For this review, take the finished solid that the model builds, in its own axes (mm). Round coordinates to 2 decimals unless told otherwise and drop trailing zeros. Use a Markdown table: item, result.
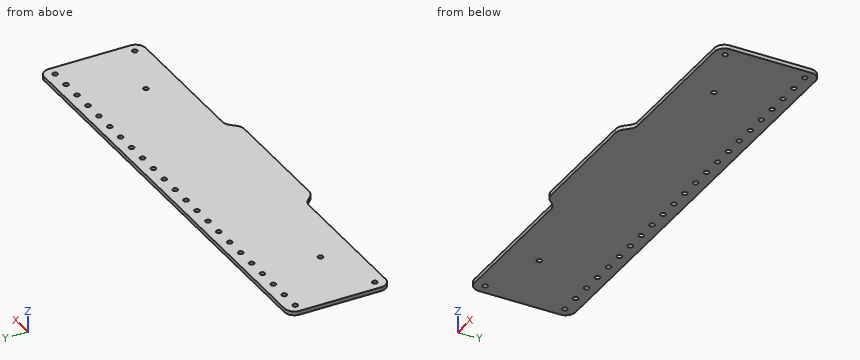
from build123d import *

# Parameters (mm, degrees)
SKETCH1_W           = 368
SKETCH1_H           = 90.35
SKETCH1_R           = 2.05
BOSS_EXTRUDE1_DEPTH = 3.175
SKETCH3_R           = 2.05
CUT_EXTRUDE1_DEPTH  = 3.18
CUT_EXTRUDE2_DEPTH  = 10
FILLET1_R           = 8


with BuildPart() as part:
    # Sketch1 → Boss-Extrude1 (new body)
    with BuildSketch(Plane.XY):
        Rectangle(SKETCH1_W, SKETCH1_H)
        with Locations((-128, -10.175)):
            Circle(SKETCH1_R, mode=Mode.SUBTRACT)
        with Locations(Location((128, -10.175, 0), (0, 0, 180))):
            Circle(SKETCH1_R, mode=Mode.SUBTRACT)
    extrude(amount=BOSS_EXTRUDE1_DEPTH)

    # Sketch3 → Cut-Extrude1 (cut)
    with BuildSketch(Plane.XY.offset(3.175)):
        with Locations((-176, 36.5)):
            Circle(SKETCH3_R)
        with Locations((-160, 36.5)):
            Circle(SKETCH3_R)
        with Locations((-144, 36.5)):
            Circle(SKETCH3_R)
        with Locations((-128, 36.5)):
            Circle(SKETCH3_R)
        with Locations((-112, 36.5)):
            Circle(SKETCH3_R)
        with Locations((-96, 36.5)):
            Circle(SKETCH3_R)
        with Locations((-80, 36.5)):
            Circle(SKETCH3_R)
        with Locations((-64, 36.5)):
            Circle(SKETCH3_R)
        with Locations((-48, 36.5)):
            Circle(SKETCH3_R)
        with Locations((-32, 36.5)):
            Circle(SKETCH3_R)
        with Locations((-16, 36.5)):
            Circle(SKETCH3_R)
        with Locations((0, 36.5)):
            Circle(SKETCH3_R)
        with Locations((16, 36.5)):
            Circle(SKETCH3_R)
        with Locations((32, 36.5)):
            Circle(SKETCH3_R)
        with Locations((48, 36.5)):
            Circle(SKETCH3_R)
        with Locations((64, 36.5)):
            Circle(SKETCH3_R)
        with Locations((80, 36.5)):
            Circle(SKETCH3_R)
        with Locations((96, 36.5)):
            Circle(SKETCH3_R)
        with Locations((112, 36.5)):
            Circle(SKETCH3_R)
        with Locations((128, 36.5)):
            Circle(SKETCH3_R)
        with Locations((144, 36.5)):
            Circle(SKETCH3_R)
        with Locations((160, 36.5)):
            Circle(SKETCH3_R)
        with Locations((176, 36.5)):
            Circle(SKETCH3_R)
        with Locations((176, -27.5)):
            Circle(SKETCH3_R)
        with Locations((-176, -27.5)):
            Circle(SKETCH3_R)
    extrude(amount=-CUT_EXTRUDE1_DEPTH, mode=Mode.SUBTRACT)

    # Sketch4 → Cut-Extrude2 (cut)
    with BuildSketch(Plane.XY.offset(3.175)):
        Polygon((-184, -36.18), (-60, -36.18), (-51.005, -45.175), (-184, -45.175), align=None)
        Polygon((184, -36.18), (184, -45.175), (51.005, -45.175), (60, -36.18), align=None)
    extrude(amount=-CUT_EXTRUDE2_DEPTH, mode=Mode.SUBTRACT)

    # Fillet1
    fillet1_edges = [part.edges().sort_by_distance(p)[0] for p in [
        (184, -36.18, 1.5875),
        (-51.005, -45.175, 1.5875),
        (-184, -36.18, 1.5875),
        (-60, -36.18, 1.5875),
        (60, -36.18, 1.5875),
        (51.005, -45.175, 1.5875),
        (-184, 45.175, 1.5875),
        (184, 45.175, 1.5875),
    ]]
    fillet(fillet1_edges, radius=FILLET1_R)


solid = part.part
Q1. Clearance check with a flat-ended pin moving along its axis: pin 1 (1 mm diameter, centred on x = -132, z = 2, fed in from -Y). State where the tip first meets the part, or that it passes through.
Determined:
| item | result |
|---|---|
| pin 1 | stops at y = -36.18 |
Q2. Wall thickness on line 1 along Y through (x, z) = (128, 1.4) (3 decimals); line 2 along X through (y, z) = (-10.5, 1.6); line 3 along Y through (x, z) = (-48, 1.9) (3 decimals): over which ranges is each line inside the solid? List them lowest first. Write a range as [from, to].
Determined:
| item | result |
|---|---|
| line 1 | y = [-36.18, -12.225], [-8.125, 34.45], [38.55, 45.175] |
| line 2 | x = [-184, -130.02], [-125.98, 125.98], [130.02, 184] |
| line 3 | y = [-45.169, 34.45], [38.55, 45.175] |
Q3. Add section A-A (z = 2.5). Give the number of separate pieces and of enclosed holes in the cut face, then the cut area to 3 significant figures.
Determined:
| item | result |
|---|---|
| separate pieces | 1 |
| enclosed holes | 27 |
| area | 30,500 mm^2 |
